CAD build for the part. Positions are in the model's coordinates, mm. Face numbers are marked on the shaded views. A direction names the side the tool comes from. Round coordinates to 2 decimals unless told otherwise and drop trailing zeros. Order: outer loops, then holes, each group sorted by start corner. A loop starts at its lowest first (then second) coordinate and runs counter-clockwise, first axis right, second up. Notation, with made-up numbers: M -31,78.25 L 20,78.25 A31 cw 20,110.25 Z; hole C 79,45 d11. An arc over 180 degrees is marked long. Put each result on its own line as item: value.
```python
from build123d import *

# Parameters (mm, degrees)
SKETCH1_R                = 20
BOSS_EXTRUDE1_DEPTH      = 17
BOSS_EXTRUDE2_DEPTH      = 20
CHAMFER1_SIZE            = 2
SKETCH3_R                = 20
BOSS_EXTRUDE3_DEPTH      = 5
FILLET1_R                = 2
CHAMFER1_OF_MIRROR1_SIZE = 2
FILLET1_OF_MIRROR1_R     = 2
SKETCH4_R                = 14.5
BOSS_EXTRUDE4_DEPTH      = 2
SKETCH5_R                = 15
BOSS_EXTRUDE5_DEPTH      = 26
SKETCH6_R                = 14.5
BOSS_EXTRUDE6_DEPTH      = 2
BOSS_EXTRUDE7_START      = 40
SKETCH7_R                = 15
BOSS_EXTRUDE7_DEPTH      = 40
FILLET2_R                = 2
CHAMFER2_SIZE            = 2
SKETCH8_R                = 17.5
BOSS_EXTRUDE8_DEPTH      = 17.5
SKETCH9_R                = 12.5
BOSS_EXTRUDE9_DEPTH      = 35
FILLET3_R                = 3
CHAMFER3_SIZE            = 2
CUT_EXTRUDE1_START       = -30
CUT_EXTRUDE1_DEPTH       = 30
CIRPATTERN1_COUNT        = 6


with BuildPart() as part:
    # Sketch1 → Boss-Extrude1 (new, symmetric)
    with BuildSketch(Plane.XY):
        Circle(SKETCH1_R)
    extrude(amount=BOSS_EXTRUDE1_DEPTH, both=True)

    # Sketch2 → Boss-Extrude2 (add)
    with BuildSketch(Plane.XY.offset(17)):
        with BuildLine():
            Line((-33.673198504, 9.545454545), (-48.104569292, -41.363636364))
            ThreePointArc((-48.104569292, -41.363636364), (0, -105), (48.104569292, -41.363636364))
            Line((48.104569292, -41.363636364), (33.673198504, 9.545454545))
            ThreePointArc((33.673198504, 9.545454545), (0, 35), (-33.673198504, 9.545454545))
        make_face()
    boss_extrude2 = extrude(amount=BOSS_EXTRUDE2_DEPTH)

    # Chamfer1
    chamfer1_edges = [part.edges().sort_by_distance(p)[0] for p in [
        (0, 35, 37),
        (-40.888883898, -15.909090909, 37),
        (0, -105, 37),
        (40.888883898, -15.909090909, 37),
    ]]
    chamfer(chamfer1_edges, length=CHAMFER1_SIZE)

    # Sketch3 → Boss-Extrude3 (add)
    with BuildSketch(Plane.XY.offset(37)):
        with Locations((0, -35)):
            Circle(SKETCH3_R)
    boss_extrude3 = extrude(amount=BOSS_EXTRUDE3_DEPTH)

    # Fillet1
    fillet1_edges = [part.edges().sort_by_distance(p)[0] for p in [
        (-20, -35, 37),
    ]]
    fillet(fillet1_edges, radius=FILLET1_R)

    # Mirror1: Boss-Extrude2, Boss-Extrude3 across plane
    add(boss_extrude2.mirror(Plane.XY))
    add(boss_extrude3.mirror(Plane.XY))

    # Chamfer1 of Mirror1
    chamfer1_of_mirror1_edges = [part.edges().sort_by_distance(p)[0] for p in [
        (0, 35, -37),
        (-40.888883898, -15.909090909, -37),
        (0, -105, -37),
        (40.888883898, -15.909090909, -37),
    ]]
    chamfer(chamfer1_of_mirror1_edges, length=CHAMFER1_OF_MIRROR1_SIZE)

    # Fillet1 of Mirror1
    fillet1_of_mirror1_edges = [part.edges().sort_by_distance(p)[0] for p in [
        (-20, -35, -37),
    ]]
    fillet(fillet1_of_mirror1_edges, radius=FILLET1_OF_MIRROR1_R)

    # Sketch4 → Boss-Extrude4 (add)
    with BuildSketch(Plane.XY.offset(42)):
        with Locations((0, -35)):
            Circle(SKETCH4_R)
    extrude(amount=BOSS_EXTRUDE4_DEPTH)

    # Sketch5 → Boss-Extrude5 (add)
    with BuildSketch(Plane.XY.offset(44)):
        with Locations(Location((0, -35, 0), (0, 0, 180))):
            Circle(SKETCH5_R)
    extrude(amount=BOSS_EXTRUDE5_DEPTH)

    # Sketch6 → Boss-Extrude6 (add)
    with BuildSketch(Plane.XY.offset(70)):
        with Locations((0, -35)):
            Circle(SKETCH6_R)
    extrude(amount=BOSS_EXTRUDE6_DEPTH)

    # Sketch7 → Boss-Extrude7 (add)
    with BuildSketch(Plane(origin=(0, 0, -42), x_dir=(-1, 0, 0), z_dir=(0, 0, -1)).offset(BOSS_EXTRUDE7_START)):
        with Locations((0, -35)):
            Circle(SKETCH7_R)
    extrude(amount=-BOSS_EXTRUDE7_DEPTH)

    # Fillet2
    fillet2_edges = [part.edges().sort_by_distance(p)[0] for p in [
        (15, -35, -42),
    ]]
    fillet(fillet2_edges, radius=FILLET2_R)

    # Chamfer2
    chamfer2_edges = [part.edges().sort_by_distance(p)[0] for p in [
        (15, -35, -82),
    ]]
    chamfer(chamfer2_edges, length=CHAMFER2_SIZE)

    # Sketch8 → Boss-Extrude8 (add)
    with BuildSketch(Plane.XY.offset(72)):
        with Locations((0, -35)):
            Circle(SKETCH8_R)
    extrude(amount=BOSS_EXTRUDE8_DEPTH)

    # Sketch9 → Boss-Extrude9 (add)
    with BuildSketch(Plane.XY.offset(89.5)):
        with Locations((0, -35)):
            Circle(SKETCH9_R)
    extrude(amount=BOSS_EXTRUDE9_DEPTH)

    # Fillet3
    fillet3_edges = [part.edges().sort_by_distance(p)[0] for p in [
        (-12.5, -35, 89.5),
    ]]
    fillet(fillet3_edges, radius=FILLET3_R)

    # Chamfer3
    chamfer3_edges = [part.edges().sort_by_distance(p)[0] for p in [
        (-12.5, -35, 124.5),
    ]]
    chamfer(chamfer3_edges, length=CHAMFER3_SIZE)

    # Sketch10 → Cut-Extrude1 (cut)
    with BuildSketch(Plane.XY.offset(124.5).offset(CUT_EXTRUDE1_START)):
        with BuildLine():
            Line((-3.454445607, -22.986807021), (-2.962947983, -24.4065615))
            ThreePointArc((-2.962947983, -24.4065615), (0, -24), (2.962947983, -24.4065615))
            Line((2.962947983, -24.4065615), (3.454445607, -22.986807021))
            ThreePointArc((3.454445607, -22.986807021), (0, -22.5), (-3.454445607, -22.986807021))
        make_face()
    cut_extrude1 = extrude(amount=CUT_EXTRUDE1_DEPTH, mode=Mode.SUBTRACT)

    # CirPattern1: Cut-Extrude1 ×6 about axis
    cirpattern1_axis = Axis((0, -35, 0), (0, 0, 1))
    for i in range(1, CIRPATTERN1_COUNT):
        add(cut_extrude1.rotate(cirpattern1_axis, i * 360 / CIRPATTERN1_COUNT), mode=Mode.SUBTRACT)


solid = part.part
```
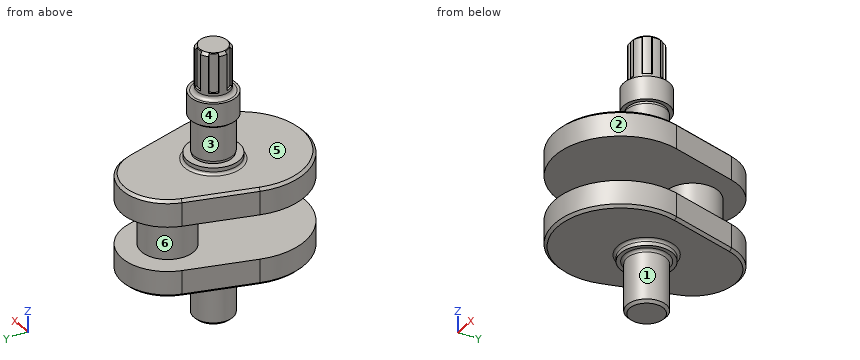
Item 1: Band-saw the part on C-C on z = 30. Give the cut face in (x, y).
Answers below:
outline: M -48.1,-41.36 A50 ccw long 48.1,-41.36 L 33.67,9.55 A35 ccw -33.67,9.55 Z
Item 2: Pin check, flat tips, straight feed: P1, Ø8, axis at y = -16.5, z = -26.5, coming from the +X side; P2, Ø10, axis at x = -6.5, y = -51.5, coming from the +Z side; P3, Ø1.3, axis at x = -9.5, y = -27.5, coming from the +Z side; P4, Ø10, axis at x = -23.5, z = 62, coming from the -Y side. Stop position of each tip, or through.
Answers below:
P1: x = 42.19
P2: z = 91.34
P3: z = 94.5
P4: through
Item 3: Probe line 1 along Z through (x, y) = (30.5, -40); line 2 along Y through (x, z) = (-0.5, 41); line 3 along Y through (x, z) = (4, 77). List the from-to ranges inside material, lowest first. Write a range as [from, to].
Answers below:
line 1: [-37, -17], [17, 37]
line 2: [-54.99, -15.01]
line 3: [-52.04, -17.96]
Item 4: Tool access for the marked faces 1, 2 and 3: list every direction of +Z, -Z, +X, -X, +Y, -Y with a clear straight run to the whole face (end or side of a thin tool).
Answers below:
face 1: -Z
face 2: +Z, -Z
face 3: none
Item 5: Band-saw the part on A-A on y = 5. Give the cut face in (x, z), and give its area (3 significant figures).
Answers below:
outline: M -34.96,-35 L -32.88,-37 L 32.88,-37 L 34.96,-35 L 34.96,-17 L 19.36,-17 L 19.36,17 L 34.96,17 L 34.96,35 L 32.88,37 L -32.88,37 L -34.96,35 L -34.96,17 L -19.36,17 L -19.36,-17 L -34.96,-17 Z
area: 4,110 mm²
Item 6: Band-saw the part on B-B on z = 53. Give the cut face in (x, y), and give its area (3 significant figures).
Answers below:
outline: C 0,-35 d30
area: 707 mm²
Item 7: Mould opens along Z. For the marked faces 4, 5 and 6 say: pulls with the +Z half, pulls with the -Z half, needs draft (parallel to the pull), parting line crosses it, or undercut.
Answers below:
face 4: needs draft
face 5: pulls with the +Z half
face 6: undercut
